```python
from build123d import *

# Parameters (mm, degrees)
F0_W      = 101.6
F0_H      = 165.1
F1_DEPTH  = 25.4
F2_W      = 77.5733087212
F2_H      = 52.7514182031
F3_DEPTH  = 61.976
F4_W      = 15.6093118712
F4_H      = 5.4604299366
F4_W_2    = 6.9440016523
F4_H_2    = 14.854170382
F4_W_3    = 25.0991685316
F4_H_3    = 15.0301940739
F4_W_4    = 6.2049590051
F4_H_4    = 14.403630048
F4_H_5    = 6.6751083359
F4_W_5    = 30.088968575
F4_H_6    = 21.6047465801
F4_H_7    = 20.752211567
F5_DEPTH  = 21.844
F6_W      = 22.5156284869
F6_H      = 54.6749219446
F6_W_2    = 23.5249437392
F6_H_2    = 57.1776889265
F7_DEPTH  = 12.7
F8_W      = 9.3237310648
F8_H      = 41.3462072611
F8_W_2    = 7.9486728646
F8_H_2    = 48.5131144524
F9_DEPTH  = 7.366
F10_R     = 3.9292089133
F11_DEPTH = 11.176


with BuildPart() as f1:
    # F0 (on Front) → F1 (new body)
    with BuildSketch(Plane.XZ):
        with Locations((-25.7154209539, -13.2609471531)):
            Rectangle(F0_W, F0_H)
    extrude(amount=F1_DEPTH)

    # F2 (on face) → F3 (cut)
    with BuildSketch(Plane.XZ.offset(25.4)):
        with Locations((-26.1394409463, 26.3757091016)):
            Rectangle(F2_W, F2_H)
    extrude(amount=-F3_DEPTH, mode=Mode.SUBTRACT)

    # F4 (on face) → F5 (join)
    with BuildSketch(Plane(origin=(0, 0, 0), x_dir=(-1, 0, 0), z_dir=(0, 1, 0))):
        with Locations((-7.8046559356, 39.4605305046)):
            Rectangle(F4_W, F4_H)
        with Locations((3.4720008262, 49.6178306639)):
            Rectangle(F4_W_2, F4_H_2)
        with Locations((3.4720008262, 39.4605305046)):
            Rectangle(F4_W_2, F4_H)
        with Locations((19.4935859181, 39.4605305046)):
            Rectangle(F4_W_3, F4_H)
        with Locations((3.4720008262, 29.2152184993)):
            Rectangle(F4_W_2, F4_H_3)
        with Locations((35.1456496865, 49.3925604969)):
            Rectangle(F4_W_4, F4_H_4)
        with Locations((35.1456496865, 39.4605305046)):
            Rectangle(F4_W_4, F4_H)
        with Locations((-7.8046559356, 18.3625672944)):
            Rectangle(F4_W, F4_H_5)
        with Locations((3.4720008262, 18.3625672944)):
            Rectangle(F4_W_2, F4_H_5)
        with Locations((53.2926134765, 39.4605305046)):
            Rectangle(F4_W_5, F4_H)
        with Locations((35.1456496865, 29.2152184993)):
            Rectangle(F4_W_4, F4_H_3)
        with Locations((19.4935859181, 18.3625672944)):
            Rectangle(F4_W_3, F4_H_5)
        with Locations((3.4720008262, 4.2226398364)):
            Rectangle(F4_W_2, F4_H_6)
        with Locations((35.1456496865, 18.3625672944)):
            Rectangle(F4_W_4, F4_H_5)
        with Locations((53.2926134765, 18.3625672944)):
            Rectangle(F4_W_5, F4_H_5)
        with Locations((35.1456496865, 4.6489073429)):
            Rectangle(F4_W_4, F4_H_7)
    extrude(amount=-F5_DEPTH)

    # F6 (on face) → F7 (cut)
    with BuildSketch(Plane.XZ.offset(25.4)):
        with Locations((-48.1722448021, -40.5984081254)):
            Rectangle(F6_W, F6_H)
        with Locations((-11.7624718696, -40.8460963517)):
            Rectangle(F6_W_2, F6_H_2)
    extrude(amount=-F7_DEPTH, mode=Mode.SUBTRACT)

    # F8 (on face) → F9 (join)
    with BuildSketch(Plane.XZ.offset(12.7)):
        with Locations((-46.2979972363, -39.0051342547)):
            Rectangle(F8_W, F8_H)
        with Locations((-9.9831267726, -40.1948392391)):
            Rectangle(F8_W_2, F8_H_2)
    extrude(amount=F9_DEPTH)

    # F10 (on face) → F11 (join)
    with BuildSketch(Plane.XZ.offset(25.4)):
        with Locations((16.8794579804, -11.9087984785)):
            Circle(F10_R)
    extrude(amount=F11_DEPTH)


solid = f1.part
```
Input: part model. Units: mm. Frame: model coordinates. A direction names the side the tool comes from. Coordinates: 2 decimals unless noted, no trailing zeros. Loops run counter-clockwise (first coordinate to the right, second up) from the corner with the lowest first, then second, coordinate; pieces in that order, holes last. Notation, with made-up numbers: M 25,30 L 84,30 A27 ccw 84,68 Z; hole C 85,1 d8. An arc over 180 degrees is marked long. Use a Markdown table: item, result. Add a question column.
1) Set-up query: faces 4 (the flat face through (-76.515, -13, -14)), 5 (the flat face through (-51, -11, 42.191)), 6 (the flat face through (-10, -20.066, -40)). Return all of +Z, -Z, +X, -X, +Y, -Y with unobstructed straight access to the full face (end or side cutting, diameter ignored); none if empty.
2) Section C-C, the plane y = -15.5. Give the number of separate pieces and of enclosed holes in the cut face, plus the area to 3 significant figures.
3) Line query: L1, parallel to X at y = -15, z = 45.5; L2, parallel to Z at x = 3.5, y = -11; L3, parallel to X at y = -25, z = -22.5. Output: solid intervals per line, ascending. Write a range as from..to.
4) Section B-B, the plane x = -21.5. Return the cut outline in (y, z).
5) Pin query (flat end, axial travel): P1, Ø3, axis at x = -19.5, z = 24, coming from the -Y side; P2, Ø8, axis at x = -63, z = -42, coming from the -Y side; P3, Ø4, axis at x = -10, z = -51.5, coming from the -Y side. Return the tip coordinate at first contact, or that it passes through.
6) Section D-D, the plane x = -34. Return the cut outline in (y, z), plus the area to 3 significant figures.
7) Draft query along Z for faces 1 (the flat face through (25.085, -13, -14)), 2 (the flat face through (-10, -16, -64.451)), 3 (the flat face through (-26, -13, 69.289)). Return one class per face: +Z half, -Z half, draft (parallel to the pull), parting line (faces both ways), or undercut.
8) Section A-A, the plane z = 27.5. Return the cut outline in (x, y), plus the area to 3 significant figures.
Answer below:
| question | item | result |
|---|---|---|
| 1 | face 4 | +Z, -Z, -X, +Y, -Y |
| 1 | face 5 | +Y, -Y |
| 1 | face 6 | -Y |
| 2 | separate pieces | 3 |
| 2 | enclosed holes | 11 |
| 2 | area | 12,400 mm2 |
| 3 | L1 | -76.52..-64.93, -38.25..-32.04, -6.94..0, 12.65..25.08 |
| 3 | L2 | -95.81..0, 15.03..21.7, 36.73..42.19, 52.75..69.29 |
| 3 | L3 | -76.52..-59.43, -36.91..-23.52, 0..25.08 |
| 4 | outline | M -25.4,-95.81 L 0,-95.81 L 0,0 L -25.4,0 L -25.4,-12.26 L -12.7,-12.26 L -12.7,-69.43 L -25.4,-69.43 Z; M -25.4,52.75 L 0,52.75 L 0,69.29 L -25.4,69.29 Z; M -21.84,15.03 L 0,15.03 L 0,21.7 L -21.84,21.7 Z; M -21.84,36.73 L 0,36.73 L 0,42.19 L -21.84,42.19 Z |
| 5 | P1 | through |
| 5 | P2 | y = -25.4 |
| 5 | P3 | y = -20.07 |
| 6 | outline | M -25.4,-95.81 L 0,-95.81 L 0,69.29 L -25.4,69.29 L -25.4,52.75 L -21.84,52.75 L -21.84,0 L -25.4,0 Z |
| 6 | area | 4,010 mm2 |
| 7 | face 1 | draft |
| 7 | face 2 | undercut |
| 7 | face 3 | +Z half |
| 8 | outline | M -76.52,-25.4 L -64.93,-25.4 L -64.93,0 L -76.52,0 Z; M -38.25,-21.84 L -32.04,-21.84 L -32.04,0 L -38.25,0 Z; M -6.94,-21.84 L 0,-21.84 L 0,0 L -6.94,0 Z; M 12.65,-25.4 L 25.08,-25.4 L 25.08,0 L 12.65,0 Z |
| 8 | area | 898 mm2 |
